from build123d import *

# Parameters (mm, degrees)
SKETCH002_R  = 1.3
PAD002_DEPTH = 7
SKETCH001_R  = 8.15
PAD001_DEPTH = 7
PAD_DEPTH    = 3


with BuildPart() as screw_holes:
    # Sketch002 → Pad002 (new body)
    with BuildSketch(Plane.XY):
        with Locations((-10, 0)):
            Circle(SKETCH002_R)
        with Locations((10, 0)):
            Circle(SKETCH002_R)
    extrude(amount=PAD002_DEPTH)


with BuildPart() as lens_hole:
    # Sketch001 → Pad001 (new body)
    with BuildSketch(Plane.XY):
        Circle(SKETCH001_R)
    extrude(amount=PAD001_DEPTH)


with BuildPart() as cut001:
    # Sketch → Pad (new body)
    with BuildSketch(Plane.XY):
        with BuildLine():
            Line((-6.5, 11), (6.5, 11))
            ThreePointArc((12.5, 5), (10.742641, 9.242641), (6.5, 11))
            Line((12.5, 5), (12.5, -5))
            ThreePointArc((6.5, -11), (10.742641, -9.242641), (12.5, -5))
            Line((6.5, -11), (-6.5, -11))
            ThreePointArc((-12.5, -5), (-10.742641, -9.242641), (-6.5, -11))
            Line((-12.5, -5), (-12.5, 5))
            ThreePointArc((-6.5, 11), (-10.742641, 9.242641), (-12.5, 5))
        make_face()
    extrude(amount=PAD_DEPTH)

    # Cut: cut Lens Hole
    add(lens_hole.part, mode=Mode.SUBTRACT)

    # Cut001: cut Screw Holes
    add(screw_holes.part, mode=Mode.SUBTRACT)


solid = cut001.part
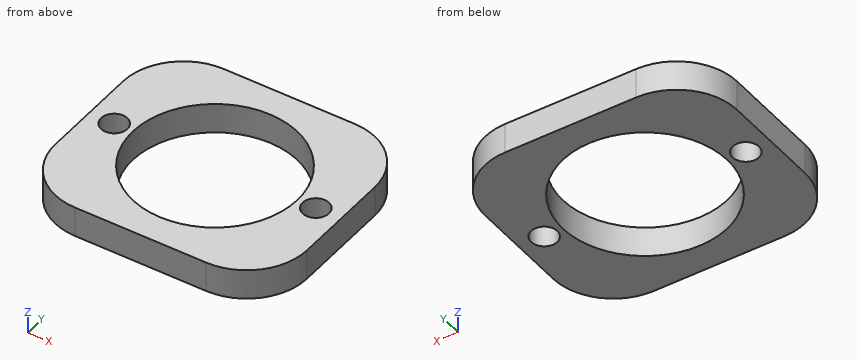
Work out the finished part from the listing and answer in its coordinate system (mm). Coordinates: 2 decimals unless noted, no trailing zeros. Write each loop counter-clockwise with the first axis right and the second up, starting at its lowest first coordinate (ties: lowest second). Pieces come first, ordered by that corner, then holes.
1. The part is cut by section D-D, the plane y = -1. Write down the section's boundary in (x, z).
Results list:
outline: (-12.5, 0) - (-10.83, 0) - (-10.83, 3) - (-12.5, 3) - close; (-9.17, 0) - (-8.09, 0) - (-8.09, 3) - (-9.17, 3) - close; (8.09, 0) - (9.17, 0) - (9.17, 3) - (8.09, 3) - close; (10.83, 0) - (12.5, 0) - (12.5, 3) - (10.83, 3) - close
2. The part is cut by section A-A, the plane z = 0.75. Write down the section's boundary in (x, y).
Results list:
outline: (-12.5, -5) arc R6 ccw to (-6.5, -11) - (6.5, -11) arc R6 ccw to (12.5, -5) - (12.5, 5) arc R6 ccw to (6.5, 11) - (-6.5, 11) arc R6 ccw to (-12.5, 5) - close; hole circle Ø2.6 at (-10, 0); hole circle Ø16.3 at (0, 0); hole circle Ø2.6 at (10, 0)
3. The part is cut by section C-C, the plane y = 3.75. Write down the section's boundary in (x, z), and give its area (3 significant figures).
Results list:
outline: (-12.5, 0) - (-7.24, 0) - (-7.24, 3) - (-12.5, 3) - close; (7.24, 0) - (12.5, 0) - (12.5, 3) - (7.24, 3) - close
area: 31.6 mm2
4. The part is cut by section B-B, the plane x = 9.75. Write down the section's boundary in (y, z), and give its area (3 significant figures).
Results list:
outline: (-10.04, 0) - (-1.28, 0) - (-1.28, 3) - (-10.04, 3) - close; (1.28, 0) - (10.04, 0) - (10.04, 3) - (1.28, 3) - close
area: 52.6 mm2
5. Consider line 1 along X through (y, z) = (0, 1.85); line 2 along Y through (x, z) = (0, 1.1); line 3 along X through (y, z) = (-7.5, 2.35). Determine where each line is inside the solid, lowest interval first.
Results list:
line 1: x = -12.5 to -11.3, -8.7 to -8.15, 8.15 to 8.7, 11.3 to 12.5
line 2: y = -11 to -8.15, 8.15 to 11
line 3: x = -11.95 to -3.19, 3.19 to 11.95
6. Flat-ended cylindrical pins translate along their axes: pin 1 (1.5 mm diameter, centred on y = -8, z = 1.5, fed in from +X); pin 2 (1.5 mm diameter, centred on x = 8, z = 2, fed in from +Y). Find the tip coordinate at first contact, or state that the pin passes through.
Results list:
pin 1: stops at x = 12.06
pin 2: stops at y = 10.95
